Geometry check sheet. Reference: the model listing, model coordinates, mm. Face numbers are marked on the shaded views. A direction names the side the tool comes from. Round coordinates to 2 decimals unless told otherwise and drop trailing zeros. Order: outer loops, then holes, each group sorted by start corner. A loop starts at its lowest first (then second) coordinate and runs counter-clockwise, first axis right, second up. Notation, with made-up numbers: (27, 73.25) -> (60, 73.25) arc R25 ccw to (60, 98.25) -> close; hole circle Ø10 at (64.5, -26.75). An arc over 180 degrees is marked (long way). Use a Markdown table: item, result. Add a question column.
Item 1: Gauge pin test, flat ends, axial feed: pin 1 Ø1 at (x, y) = (-68.5, 2.5) entering from -Z; pin 2 Ø4 at (x, y) = (-22, 48.5) entering from -Z; pin 3 Ø1 at (x, y) = (-50.5, 41) entering from -Z. Record the tip position at first contact, or that the pin passes through.
Item 2: Set-up check for the marked faces 1 and 2: record each of +Z, -Z, +X, -X, +Y, -Y from which the full face is reachable in a straight line by a thin tool's end or side.
Item 3: Sectioned sample at C-C, the plane z = -32. Record the cut outline in (x, y).
Item 4: Material ranges on probe 1 along Z at (x, y) = (-74.5, 41); probe 2 along Z at (x, y) = (0, 19), recorded low to high. Write a range as [from, to].
Item 5: Sectioned sample at B-B, the plane x = -44. Record the cut outline in (y, z), and give its area (3 significant figures).
Item 6: Sectioned sample at D-D, the plane x = 9.5. Record the cut outline in (y, z).
from build123d import *

# Parameters (mm, degrees)
SKETCH1_R           = 4.28625
BOSS_EXTRUDE1_DEPTH = 50.8
FILLET2_R           = 2.54
SKETCH7_W           = 44.675933609
SKETCH7_H           = 44.675933609
CUT_EXTRUDE3_DEPTH  = 3.429
FILLET9_R           = 3.175
BOSS_EXTRUDE2_DEPTH = 30.1625
CUT_EXTRUDE4_START  = -4.7625
CUT_EXTRUDE4_DEPTH  = 4.7625


with BuildPart() as part:
    # Sketch1 → Boss-Extrude1 (new body)
    with BuildSketch(Plane(origin=(0, 0, 0), x_dir=(1, 0, 0), z_dir=(0, 1, 0))):
        with BuildLine():
            Line((13.462, 57.17106993), (-10.037787665, 10.037787665))
            Line((-10.037787665, 10.037787665), (-57.17106993, -13.462))
            Line((-57.17106993, -13.462), (-127, -13.462))
            Line((-127, -13.462), (-127, -18.542))
            Line((-127, -18.542), (0, -18.542))
            ThreePointArc((0, -18.542), (13.111173937, -13.111173937), (18.542, 0))
            Line((18.542, 0), (18.542, 127))
            Line((18.542, 127), (13.462, 127))
            Line((13.462, 127), (13.462, 57.17106993))
        make_face()
        with Locations(Location((0, 0, 0), (0, 0, 270))):
            Circle(SKETCH1_R, mode=Mode.SUBTRACT)
    extrude(amount=BOSS_EXTRUDE1_DEPTH)

    # Fillet2
    fillet2_edges = [part.edges().sort_by_distance(p)[0] for p in [
        (13.462, 25.4, -127),
        (18.542, 25.4, -127),
        (-127, 25.4, 13.462),
        (-127, 25.4, 18.542),
    ]]
    fillet(fillet2_edges, radius=FILLET2_R - 0.0001)  # a hair under: the kernel refuses the full size

    # Sketch7 → Cut-Extrude3 (cut)
    with BuildSketch(Plane(origin=(0, 50.8, 0), x_dir=(1, 0, 0), z_dir=(0, 1, 0))):
        with Locations((-17.511966805, 17.511966805)):
            Rectangle(SKETCH7_W, SKETCH7_H)
    extrude(amount=-CUT_EXTRUDE3_DEPTH, mode=Mode.SUBTRACT)

    # Fillet9
    fillet9_edges = [part.edges().sort_by_distance(p)[0] for p in [
        (4.826, 49.0855, -39.849933609),
        (4.826, 49.0855, 4.826),
        (-39.849933609, 49.0855, 4.826),
    ]]
    fillet(fillet9_edges, radius=FILLET9_R)

    # Sketch8 → Boss-Extrude2 (add, symmetric)
    with BuildSketch(Plane(origin=(0, 25.4, 0), x_dir=(1, 0, 0), z_dir=(0, 1, 0))):
        with BuildLine():
            Line((0, -13.462), (-124.46, -13.462))
            ThreePointArc((-124.46, -13.462), (-126.256051224, -14.205948776), (-127, -16.002))
            ThreePointArc((-127, -16.002), (-126.256051224, -17.798051224), (-124.46, -18.542))
            Line((-124.46, -18.542), (0, -18.542))
            ThreePointArc((0, -18.542), (13.111173937, -13.111173937), (18.542, 0))
            Line((18.542, 0), (18.542, 124.46))
            ThreePointArc((18.542, 124.46), (17.798051224, 126.256051224), (16.002, 127))
            ThreePointArc((16.002, 127), (14.205948776, 126.256051224), (13.462, 124.46))
            Line((13.462, 124.46), (13.462, 0))
            ThreePointArc((13.462, 0), (9.519071488, -9.519071488), (0, -13.462))
        make_face()
    extrude(amount=BOSS_EXTRUDE2_DEPTH, both=True)

    # Sketch9 → Cut-Extrude4 (cut)
    with BuildSketch(Plane.XZ.offset(4.7625).offset(CUT_EXTRUDE4_START)):
        with BuildLine():
            Line((7.112, 13.462), (0, 13.462))
            ThreePointArc((0, 13.462), (9.519071488, 9.519071488), (13.462, 0))
            Line((13.462, 0), (13.462, 7.112))
            ThreePointArc((13.462, 7.112), (11.602128061, 11.602128061), (7.112, 13.462))
        make_face()
    extrude(amount=CUT_EXTRUDE4_DEPTH, mode=Mode.SUBTRACT)


solid = part.part
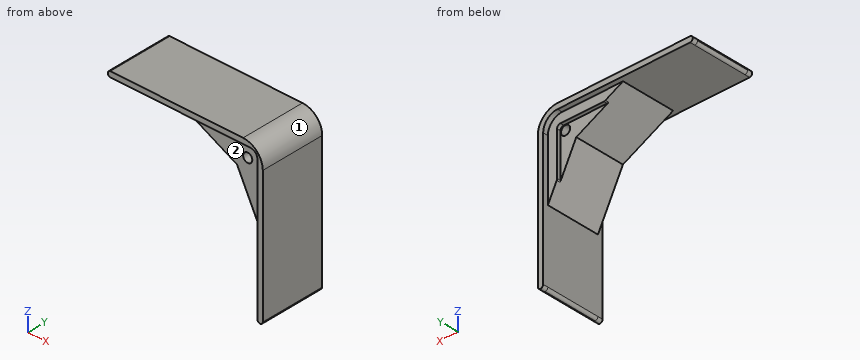
Found:
| question | item | result |
|---|---|---|
| 1 | pin 1 | stops at z = 13.46 |
| 1 | pin 2 | stops at z = -4.9 |
| 1 | pin 3 | stops at z = 9.89 |
| 2 | face 1 | +Z, +X, +Y, -Y |
| 2 | face 2 | -Z, -X, -Y |
| 3 | outline | (0.91, 0) -> (13.46, 0) -> (13.46, -4.76) -> (18.54, -4.76) -> (18.54, 55.56) -> (13.46, 55.56) -> (13.46, 50.8) -> (4.83, 50.8) -> (4.83, 47.37) -> (0.91, 47.37) -> close |
| 4 | probe 1 | z = [13.46, 18.54] |
| 4 | probe 2 | z = [-30.17, -4.29], [4.29, 18.54] |
| 5 | outline | (-4.76, 13.46) -> (0, 13.46) -> (0, 6.9) -> (50.8, 6.9) -> (50.8, 13.46) -> (55.56, 13.46) -> (55.56, 18.54) -> (-4.76, 18.54) -> close |
| 5 | area | 640 mm2 |
| 6 | outline | (-4.76, 13) -> (0, 13) -> (0, -49.22) -> (50.8, -49.22) -> (50.8, 9.54) -> (55.56, 9.54) -> (55.56, 15.92) -> (-4.76, 15.92) -> close |
